from build123d import *

# Parameters (mm, degrees)
SKETCH_1_W          = 50
SKETCH_1_H          = 38
SKETCH_1_R          = 1.0000000000000018
SKETCH_1_R_2        = 1.0000000000000016
EXTRUDE_1_DEPTH     = 2
EXTRUDE_2_DEPTH     = 3
SKETCH_5_W          = 24
SKETCH_5_H          = 26
CUT_EXTRUDE_1_DEPTH = 33.66496594212216
FILLET_1_R          = 2
EXTRUDE_6_DEPTH     = 2
CUT_EXTRUDE_2_REACH = 38.993
FILLET_2_R          = 1
CUT_EXTRUDE_3_REACH = 37.814
SKETCH_8_R          = 1.6
SKETCH_8_R_2        = 1.6000000000000019


with BuildPart() as part:
    # 草图1 → 凸台-拉伸1 (new body)
    with BuildSketch(Plane(origin=(0, 0, 0), x_dir=(1, 0, 0), z_dir=(0, 1, 0))):
        Rectangle(SKETCH_1_W, SKETCH_1_H)
        with Locations(Location((-22.600000000000005, 16.500000000000004, 0), (0, 0, 270))):
            Circle(SKETCH_1_R, mode=Mode.SUBTRACT)
        with Locations(Location((-22.600000000000005, -1.4999999999999944, 0), (0, 0, 270))):
            Circle(SKETCH_1_R_2, mode=Mode.SUBTRACT)
        with Locations(Location((22.599999999999998, 16.500000000000004, 0), (0, 0, 270))):
            Circle(SKETCH_1_R, mode=Mode.SUBTRACT)
        with Locations(Location((22.599999999999998, -1.4999999999999944, 0), (0, 0, 270))):
            Circle(SKETCH_1_R_2, mode=Mode.SUBTRACT)
    extrude(amount=EXTRUDE_1_DEPTH)

    # 草图3 → 凸台-拉伸2 (add)
    with BuildSketch(Plane(origin=(12, 0, 0), x_dir=(0, 0, -1), z_dir=(1, 0, 0))):
        Polygon((-18.999999999999996, -2), (-10.339745962155614, -7.000000000000011), (19.000000000000004, 0), (-18.999999999999996, 0), align=None)
    extrude_2 = extrude(amount=EXTRUDE_2_DEPTH)

    # 镜向1: 凸台-拉伸2 across plane
    add(extrude_2.mirror(Plane(origin=(0, 0, 0), x_dir=(0, 0, 1), z_dir=(1, 0, 0))))

    # 草图5 → 切除-拉伸1 (cut, through all)
    with BuildSketch(Plane(origin=(0, 2, 0), x_dir=(1, 0, 0), z_dir=(0, 1, 0))):
        with Locations((0, -5.9999999999999964)):
            Rectangle(SKETCH_5_W, SKETCH_5_H)
    extrude(amount=-CUT_EXTRUDE_1_DEPTH, mode=Mode.SUBTRACT)

    # 圆角1
    fillet_1_edges = [part.edges().sort_by_distance(p)[0] for p in [
        (12, 1, -7.000000000000003),
        (-12, 1, -7.000000000000003),
        (25.000000000000004, 1, 18.999999999999996),
        (-24.999999999999996, 1, 18.999999999999996),
        (-24.999999999999996, 1, -19.000000000000004),
        (25.000000000000004, 1, -19.000000000000004),
    ]]
    fillet(fillet_1_edges, radius=FILLET_1_R)

    # 草图6 → 凸台-拉伸6 (add)
    with BuildSketch(Plane(origin=(0, -9.72724133595218, 5.616025403784458), x_dir=(1, 0, 0), z_dir=(0, -0.866025403784438, 0.5000000000000011))):
        Polygon((-15, 15.45448267190432), (15, 15.45448267190432), (15, -0.5455173280956814), (-14.999999999999998, -0.5455173280956814), align=None)
    extrude(amount=-EXTRUDE_6_DEPTH)

    # 草图7 → 切除-拉伸2 (cut, up to next)
    with BuildSketch(Plane(origin=(0, -9.72724133595218, 5.616025403784458), x_dir=(1, 0, 0), z_dir=(0, -0.866025403784438, 0.5000000000000011)), mode=Mode.PRIVATE) as cut_extrude_2_sk1:
        with BuildLine():
            Line((-14.999999999999998, -0.5455173280956823), (15, -0.5455173280956823))
            Line((15, -0.5455173280956823), (14.999999999999996, 0.45448267190431774))
            ThreePointArc((14.999999999999996, 0.45448267190431774), (-3.22e-15, 7.225726116581361), (-14.999999999999998, 0.454482671904316))
            Line((-14.999999999999998, 0.454482671904316), (-14.999999999999998, -0.5455173280956823))
        make_face()
    cut_extrude_2_tool1 = extrude(cut_extrude_2_sk1.sketch, amount=-CUT_EXTRUDE_2_REACH, mode=Mode.PRIVATE) & part.part
    add(cut_extrude_2_tool1.solids().sort_by_distance((0, -8.409568, 7.898302))[0], mode=Mode.SUBTRACT)

    # 圆角2
    fillet_2_edges = [part.edges().sort_by_distance(p)[0] for p in [
        (-12, -1.133974596215562, 18.499999999999996),
        (12, -1.1339745962155647, 18.499999999999993),
        (14.999999999999996, -8.63397459621558, 5.5096189432334235),
        (-15, -8.633974596215584, 5.509618943233422),
    ]]
    fillet(fillet_2_edges, radius=FILLET_2_R)

    # 草图8 → 切除-拉伸3 (cut, up to next)
    with BuildSketch(Plane(origin=(0, -7.9951905283833, 4.616025403784459), x_dir=(1, 0, 0), z_dir=(0, 0.866025403784438, -0.5000000000000012)), mode=Mode.PRIVATE) as cut_extrude_3_sk1:
        with Locations(Location((-5.999999999999998, -11.454482671904318, 0), (0, 0, 270))):
            Circle(SKETCH_8_R)
    cut_extrude_3_tool1 = extrude(cut_extrude_3_sk1.sketch, amount=-CUT_EXTRUDE_3_REACH, mode=Mode.PRIVATE) & part.part
    # 草图8 → 切除-拉伸3 (cut, up to next)
    with BuildSketch(Plane(origin=(0, -7.9951905283833, 4.616025403784459), x_dir=(1, 0, 0), z_dir=(0, 0.866025403784438, -0.5000000000000012)), mode=Mode.PRIVATE) as cut_extrude_3_sk2:
        with Locations(Location((6.000000000000002, -11.454482671904316, 0), (0, 0, 270))):
            Circle(SKETCH_8_R_2)
    cut_extrude_3_tool2 = extrude(cut_extrude_3_sk2.sketch, amount=-CUT_EXTRUDE_3_REACH, mode=Mode.PRIVATE) & part.part
    add(cut_extrude_3_tool1.solids().sort_by_distance((-6, -2.267949, 14.535898))[0], mode=Mode.SUBTRACT)
    add(cut_extrude_3_tool2.solids().sort_by_distance((6, -2.267949, 14.535898))[0], mode=Mode.SUBTRACT)


solid = part.part
The listing builds one solid part. Answer for the finished solid, in the listing's coordinates (mm). A direction names the side the tool comes from. Give positions to 0.01 mm unless a question says otherwise; leave off trailing zeros. Write each loop counter-clockwise with the first axis right and the second up, starting at its lowest first coordinate (ties: lowest second). Pieces come first, ordered by that corner, then holes.
1) Section C-C (x = 0) is taken. Write down the section's boundary in (y, z), and give its area (3 significant figures).
2) For a pull along X with two mould halves and no side action, classify faces 1 (the face through (-21.76, 0.99, -15.96)), 2 (the face through (-24.43, 1.01, -18.4)), 3 (the face through (13.479, -3.207, -5.56)), 4 (the face through (23.44, 0.99, 2.04)) as pulls with the +X half, pulls with the -X half, needs draft (parallel to the pull), parting line crosses it, or undercut.
3) Section B-B (z = -4) is taken. Write down the section's boundary in (x, y), and give its area (3 significant figures).
4) Given P1, Ø2.5, axis at y = -3, z = -6.5, coming from the +X side; P2, Ø2.5, axis at x = -22.6, z = 1.5, coming from the -Y side; P3, Ø3, axis at x = 2.5, y = -4.5, coming from the -Z side; P4, Ø6, axis at y = -6.5, z = -11.5, coming from the +X side, each flat-ended and moving along its own axis, determine where each tip first touches the part or whether it passes through.
5) Section D-D (z = 1.5) is taken. Write down the section's boundary in (x, y).
6) A tool of negligible diameter and unlimited length cuts with its end or side. For faces 5 (the face through (20, 0, 0)), 6 (the face through (-15, -2, 4)), 7 (the face through (-11.56, -0.84, 18.53)), from which of +Z, -Z, +X, -X, +Y, -Y can it reach the whole face along a straight path? Write none if from no direction.
7) Find the intervals of material crossed by L1, parallel to X at y = 1.15, z = 1.5; L2, parallel to X at y = 0.5, z = -16.5; L3, parallel to Z at x = 22.6, y = 0.75, in increasing order.
8) Section A-A (y = 0.75) is taken. Write down the section's boundary in (x, z), and give its area (3 significant figures).
Response:
1. outline: (-6.11, 11.87) - (-4.38, 10.87) - (-0.27, 18) - (-2, 19) - close; (0, -19) - (2, -19) - (2, -7) - (0, -7) - close
1. area: 40.5 mm2
2. face 1: undercut
2. face 2: pulls with the -X half
2. face 3: needs draft
2. face 4: undercut
3. outline: (-25, 0) - (-15, 0) - (-15, -3.58) - (-12, -3.58) - (-12, 2) - (-25, 2) - close; (12, -3.58) - (15, -3.58) - (15, 0) - (25, 0) - (25, 2) - (12, 2) - close
3. area: 73.5 mm2
4. P1: stops at x = 15
4. P2: stops at y = 0
4. P3: stops at z = 10.52
4. P4: passes through
5. outline: (-25, 0) - (-23.6, 0) - (-23.6, 2) - (-25, 2) - close; (-21.6, 0) - (-15, 0) - (-15, -4.89) - (-12, -4.89) - (-12, 2) - (-21.6, 2) - close; (12, -4.89) - (15, -4.89) - (15, 0) - (21.6, 0) - (21.6, 2) - (12, 2) - close; (23.6, 0) - (25, 0) - (25, 2) - (23.6, 2) - close
6. face 5: +Z, -Z, +X, -Y
6. face 6: +Z, -Z, -X, -Y
6. face 7: +Z, +Y
7. L1: x = -25 to -23.6, -21.6 to -12, 12 to 21.6, 23.6 to 25
7. L2: x = -25 to -23.6, -21.6 to 21.6, 23.6 to 25
7. L3: z = -19 to -17.5, -15.5 to 0.5, 2.5 to 19
8. outline: (-25, -17) arc R2 ccw to (-23, -19) - (23, -19) arc R2 ccw to (25, -17) - (25, 17) arc R2 ccw to (23, 19) - (12, 19) - (12, -5) arc R2 cw to (10, -7) - (-10, -7) arc R2 cw to (-12, -5) - (-12, 19) - (-23, 19) arc R2 ccw to (-25, 17) - close; hole circle Ø2 at (-22.6, -16.5); hole circle Ø2 at (-22.6, 1.5); hole circle Ø2 at (22.6, -16.5); hole circle Ø2 at (22.6, 1.5)
8. area: 1,260 mm2
